Design review of the part built by this model. Coordinates are the model's own, in mm. A direction names the side the tool comes from. Give positions to 0.01 mm unless a question says otherwise; leave off trailing zeros. Return JSON: item names as keys, results as strings.
```python
from build123d import *

# Parameters (mm, degrees)
F0_R     = 14.2875
F0_R_2   = 10.9601
F1_DEPTH = 3.175
F3_DEPTH = 3.175


with BuildPart() as f1:
    # F0 (on Front) → F1 (new body)
    with BuildSketch(Plane.XZ):
        Circle(F0_R)
        Circle(F0_R_2, mode=Mode.SUBTRACT)
    extrude(amount=F1_DEPTH)

    # F2 (on Front) → F3 (join, through all)
    with BuildSketch(Plane.XZ):
        with BuildLine():
            Line((0, 14.266242), (-0.433452, 15.106783))
            ThreePointArc((-0.433452, 15.106783), (-1.019514, 15.078573), (-1.604039, 15.027635))
            Line((-1.604039, 15.027635), (-1.897302, 14.050528))
            Line((-1.897302, 14.050528), (0, 14.266242))
        make_face()
        with BuildLine():
            ThreePointArc((-3.564857, 14.686544), (-4.132247, 14.537101), (-4.693408, 14.365747))
            Line((-4.693408, 14.365747), (-4.777111, 13.349018))
            Line((-4.777111, 13.349018), (-2.966118, 13.95449))
            Line((-2.966118, 13.95449), (-3.564857, 14.686544))
        make_face()
        with BuildLine():
            ThreePointArc((-6.54046, 13.624432), (-7.06438, 13.360288), (-7.577653, 13.076007))
            Line((-7.577653, 13.076007), (-7.448136, 12.064093))
            Line((-7.448136, 12.064093), (-5.802603, 13.03286))
            Line((-5.802603, 13.03286), (-6.54046, 13.624432))
        make_face()
        with BuildLine():
            ThreePointArc((-9.230214, 11.966867), (-9.687767, 11.599566), (-10.130717, 11.214782))
            Line((-10.130717, 11.214782), (-9.793643, 10.251909))
            Line((-9.793643, 10.251909), (-8.385486, 11.541632))
            Line((-8.385486, 11.541632), (-9.230214, 11.966867))
        make_face()
        with BuildLine():
            ThreePointArc((-11.516564, 9.786293), (-11.887751, 9.331888), (-12.241021, 8.863418))
            Line((-12.241021, 8.863418), (-11.71112, 7.991668))
            Line((-11.71112, 7.991668), (-10.601884, 9.545979))
            Line((-10.601884, 9.545979), (-11.516564, 9.786293))
        make_face()
        with BuildLine():
            ThreePointArc((-13.299584, 7.178011), (-13.568184, 6.656362), (-13.816334, 6.124679))
            Line((-13.816334, 6.124679), (-13.116765, 5.382152))
            Line((-13.116765, 5.382152), (-12.354928, 7.133121))
            Line((-12.354928, 7.133121), (-13.299584, 7.178011))
        make_face()
        with BuildLine():
            ThreePointArc((-14.501348, 4.256015), (-14.655622, 3.68992), (-14.787806, 3.118263))
            Line((-14.787806, 3.118263), (-13.949144, 2.53741))
            Line((-13.949144, 2.53741), (-13.568002, 4.408511))
            Line((-13.568002, 4.408511), (-14.501348, 4.256015))
        make_face()
        with BuildLine():
            ThreePointArc((-15.069334, 1.148011), (-15.102539, 0.562211), (-15.11298, -0.024436))
            Line((-15.11298, -0.024436), (-14.171879, -0.418229))
            Line((-14.171879, -0.418229), (-14.18809, 1.491228))
            Line((-14.18809, 1.491228), (-15.069334, 1.148011))
        make_face()
        with BuildLine():
            ThreePointArc((-14.978718, -2.010166), (-14.889403, -2.590069), (-14.777645, -3.166068))
            Line((-14.777645, -3.166068), (-13.775235, -3.355589))
            Line((-13.775235, -3.355589), (-14.18809, -1.491228))
            Line((-14.18809, -1.491228), (-14.978718, -2.010166))
        make_face()
        with BuildLine():
            ThreePointArc((-14.23346, -5.08049), (-14.025528, -5.629151), (-13.796455, -6.169326))
            Line((-13.796455, -6.169326), (-12.776547, -6.146293))
            Line((-12.776547, -6.146293), (-13.568002, -4.408511))
            Line((-13.568002, -4.408511), (-14.23346, -5.08049))
        make_face()
        with BuildLine():
            ThreePointArc((-12.866132, -7.928772), (-12.54867, -8.422211), (-12.212295, -8.902956))
            Line((-12.212295, -8.902956), (-11.219463, -8.668376))
            Line((-11.219463, -8.668376), (-12.354928, -7.133121))
            Line((-12.354928, -7.133121), (-12.866132, -7.928772))
        make_face()
        with BuildLine():
            ThreePointArc((-10.936491, -10.430528), (-10.523375, -10.847181), (-10.094398, -11.247484))
            Line((-10.094398, -11.247484), (-9.172034, -10.811608))
            Line((-9.172034, -10.811608), (-10.601884, -9.545979))
            Line((-10.601884, -9.545979), (-10.936491, -10.430528))
        make_face()
        with BuildLine():
            ThreePointArc((-8.528874, -12.476421), (-8.038159, -12.798077), (-7.535328, -13.100443))
            Line((-7.535328, -13.100443), (-6.723743, -12.482322))
            Line((-6.723743, -12.482322), (-8.385486, -11.541632))
            Line((-8.385486, -11.541632), (-8.528874, -12.476421))
        make_face()
        with BuildLine():
            ThreePointArc((-5.748504, -13.977034), (-5.201636, -14.189635), (-4.646927, -14.38085))
            Line((-4.646927, -14.38085), (-3.981593, -13.607498))
            Line((-3.981593, -13.607498), (-5.802603, -13.03286))
            Line((-5.802603, -13.03286), (-5.748504, -13.977034))
        make_face()
        with BuildLine():
            ThreePointArc((-2.716897, -14.866783), (-2.137777, -14.961039), (-1.555434, -15.032744))
            Line((-1.555434, -15.032744), (-1.065427, -14.137961))
            Line((-1.065427, -14.137961), (-2.966118, -13.95449))
            Line((-2.966118, -13.95449), (-2.716897, -14.866783))
        make_face()
        with BuildLine():
            ThreePointArc((0.433452, -15.106783), (1.019514, -15.078573), (1.604039, -15.027635))
            Line((1.604039, -15.027635), (1.897302, -14.050528))
            Line((1.897302, -14.050528), (0, -14.266242))
            Line((0, -14.266242), (0.433452, -15.106783))
        make_face()
        with BuildLine():
            ThreePointArc((3.564857, -14.686544), (4.132247, -14.537101), (4.693408, -14.365747))
            Line((4.693408, -14.365747), (4.777111, -13.349018))
            Line((4.777111, -13.349018), (2.966118, -13.95449))
            Line((2.966118, -13.95449), (3.564857, -14.686544))
        make_face()
        with BuildLine():
            ThreePointArc((6.54046, -13.624432), (7.06438, -13.360288), (7.577653, -13.076007))
            Line((7.577653, -13.076007), (7.448136, -12.064093))
            Line((7.448136, -12.064093), (5.802603, -13.03286))
            Line((5.802603, -13.03286), (6.54046, -13.624432))
        make_face()
        with BuildLine():
            ThreePointArc((9.230214, -11.966867), (9.687767, -11.599566), (10.130717, -11.214782))
            Line((10.130717, -11.214782), (9.793643, -10.251909))
            Line((9.793643, -10.251909), (8.385486, -11.541632))
            Line((8.385486, -11.541632), (9.230214, -11.966867))
        make_face()
        with BuildLine():
            ThreePointArc((11.516564, -9.786293), (11.887751, -9.331888), (12.241021, -8.863418))
            Line((12.241021, -8.863418), (11.71112, -7.991668))
            Line((11.71112, -7.991668), (10.601884, -9.545979))
            Line((10.601884, -9.545979), (11.516564, -9.786293))
        make_face()
        with BuildLine():
            ThreePointArc((13.299584, -7.178011), (13.568184, -6.656362), (13.816334, -6.124679))
            Line((13.816334, -6.124679), (13.116765, -5.382152))
            Line((13.116765, -5.382152), (12.354928, -7.133121))
            Line((12.354928, -7.133121), (13.299584, -7.178011))
        make_face()
        with BuildLine():
            ThreePointArc((14.501348, -4.256015), (14.655622, -3.68992), (14.787806, -3.118263))
            Line((14.787806, -3.118263), (13.949144, -2.53741))
            Line((13.949144, -2.53741), (13.568002, -4.408511))
            Line((13.568002, -4.408511), (14.501348, -4.256015))
        make_face()
        with BuildLine():
            ThreePointArc((15.069334, -1.148011), (15.102539, -0.562211), (15.11298, 0.024436))
            Line((15.11298, 0.024436), (14.171879, 0.418229))
            Line((14.171879, 0.418229), (14.18809, -1.491228))
            Line((14.18809, -1.491228), (15.069334, -1.148011))
        make_face()
        with BuildLine():
            ThreePointArc((14.978718, 2.010166), (14.889403, 2.590069), (14.777645, 3.166068))
            Line((14.777645, 3.166068), (13.775235, 3.355589))
            Line((13.775235, 3.355589), (14.18809, 1.491228))
            Line((14.18809, 1.491228), (14.978718, 2.010166))
        make_face()
        with BuildLine():
            ThreePointArc((14.23346, 5.08049), (14.025528, 5.629151), (13.796455, 6.169326))
            Line((13.796455, 6.169326), (12.776547, 6.146293))
            Line((12.776547, 6.146293), (13.568002, 4.408511))
            Line((13.568002, 4.408511), (14.23346, 5.08049))
        make_face()
        with BuildLine():
            ThreePointArc((12.866132, 7.928772), (12.54867, 8.422211), (12.212295, 8.902956))
            Line((12.212295, 8.902956), (11.219463, 8.668376))
            Line((11.219463, 8.668376), (12.354928, 7.133121))
            Line((12.354928, 7.133121), (12.866132, 7.928772))
        make_face()
        with BuildLine():
            ThreePointArc((10.936491, 10.430528), (10.523375, 10.847181), (10.094398, 11.247484))
            Line((10.094398, 11.247484), (9.172034, 10.811608))
            Line((9.172034, 10.811608), (10.601884, 9.545979))
            Line((10.601884, 9.545979), (10.936491, 10.430528))
        make_face()
        with BuildLine():
            ThreePointArc((8.528874, 12.476421), (8.038159, 12.798077), (7.535328, 13.100443))
            Line((7.535328, 13.100443), (6.723743, 12.482322))
            Line((6.723743, 12.482322), (8.385486, 11.541632))
            Line((8.385486, 11.541632), (8.528874, 12.476421))
        make_face()
        with BuildLine():
            ThreePointArc((5.748504, 13.977034), (5.201636, 14.189635), (4.646927, 14.38085))
            Line((4.646927, 14.38085), (3.981593, 13.607498))
            Line((3.981593, 13.607498), (5.802603, 13.03286))
            Line((5.802603, 13.03286), (5.748504, 13.977034))
        make_face()
        with BuildLine():
            ThreePointArc((2.716897, 14.866783), (2.137777, 14.961039), (1.555434, 15.032744))
            Line((1.555434, 15.032744), (1.065427, 14.137961))
            Line((1.065427, 14.137961), (2.966118, 13.95449))
            Line((2.966118, 13.95449), (2.716897, 14.866783))
        make_face()
    extrude(amount=F3_DEPTH)


solid = f1.part
```
Item 1: Mouldability with a two-part tool opening along Z and no side actions: class faces 1 (the face through (10.53, -1.57, 10.84)), 2 (the face through (-5.775, -1.565, -13.51)), 3 (the face through (-8.458, -1.565, -12.014)) as released by +Z, released by -Z, zero draft, split by the parting line, or undercut.
Result set:
{"face 1": "released by +Z", "face 2": "released by -Z", "face 3": "undercut"}
Item 2: Machinability: for faces 4 (the face through (8.458, -1.565, 12.014)), 5 (the face through (-14.257, -1.565, -0.931)), 6 (the face through (11.88, -1.57, -9.34)), which of the approach directions +Z, -Z, +X, -X, +Y, -Y give a long, thin tool a straight path to every point of the face, cutting with its end or side? Answer none if there is none.
Result set:
{"face 4": "+X, +Y, -Y", "face 5": "-X, +Y, -Y", "face 6": "-Z, +X, +Y, -Y"}
Item 3: For pin 1 (1 mm diameter, centred on x = -2.5, z = -8.5, fed in from -Y) (3 decimals); pin 2 (1.5 mm diameter, centred on y = -1, z = -10, fed in from +X), all flat-tipped, find the tip position at first contact; note any pin that passes through.
Result set:
{"pin 1": "passes through", "pin 2": "stops at x = 11.95"}
Item 4: Wall thickness on L1, parallel to Z at x = 5, y = -2.75; L2, parallel to Z at x = -6, y = -0.45; L3, parallel to X at y = -1.55, z = 10: over which ranges is each line inside the solid? List them lowest first. Write a range as [from, to].
Result set:
{"L1": "z = [-13.38, -9.75], [9.75, 14.26]", "L2": "z = [-12.97, -9.17], [9.17, 13.19]", "L3": "x = [-10.2, -4.49], [4.49, 10.77]"}
